from build123d import *

# Parameters (mm, degrees)
ESQUISSE1_W             = 100
ESQUISSE1_H             = 150
BOSS_EXTRU_1_DEPTH      = 100
ESQUISSE2_W             = 90
ESQUISSE2_H             = 140
ENL_V_MAT_EXTRU_1_DEPTH = 95
ESQUISSE4_W             = 40
ESQUISSE4_H             = 150
BOSS_EXTRU_2_DEPTH      = 10
ESQUISSE5_W             = 6
ESQUISSE5_H             = 150
ENL_V_MAT_EXTRU_2_DEPTH = 5
ESQUISSE7_W             = 40
ESQUISSE7_H             = 150
BOSS_EXTRU_3_DEPTH      = 10
ESQUISSE8_W             = 6
ESQUISSE8_H             = 150
ENL_V_MAT_EXTRU_3_DEPTH = 5
ESQUISSE9_W             = 5
ESQUISSE9_H             = 5
ENL_V_MAT_EXTRU_4_DEPTH = 121
ESQUISSE10_W            = 2.816855809
ESQUISSE10_H            = 20
BOSS_EXTRU_4_DEPTH      = 20
ESQUISSE11_R            = 4
ENL_V_MAT_EXTRU_5_DEPTH = 111


with BuildPart() as part:
    # Esquisse1 → Boss.-Extru.1 (new body)
    with BuildSketch(Plane.XY):
        with Locations((50, 75)):
            Rectangle(ESQUISSE1_W, ESQUISSE1_H)
    extrude(amount=BOSS_EXTRU_1_DEPTH)

    # Esquisse2 → Enlèv. mat.-Extru.1 (cut)
    with BuildSketch(Plane(origin=(0, 0, 0), x_dir=(-1, 0, 0), z_dir=(0, 0, -1))):
        with Locations((-50, 75)):
            Rectangle(ESQUISSE2_W, ESQUISSE2_H)
    extrude(amount=-ENL_V_MAT_EXTRU_1_DEPTH, mode=Mode.SUBTRACT)

    # Esquisse4 → Boss.-Extru.2 (add)
    with BuildSketch(Plane.ZY):
        with Locations((50, 75)):
            Rectangle(ESQUISSE4_W, ESQUISSE4_H)
    extrude(amount=BOSS_EXTRU_2_DEPTH)

    # Esquisse5 → Enlèv. mat.-Extru.2 (cut)
    with BuildSketch(Plane.ZY.offset(10)):
        with Locations((50, 75)):
            Rectangle(ESQUISSE5_W, ESQUISSE5_H)
    extrude(amount=-ENL_V_MAT_EXTRU_2_DEPTH, mode=Mode.SUBTRACT)

    # Esquisse7 → Boss.-Extru.3 (add)
    with BuildSketch(Plane(origin=(100, 0, 0), x_dir=(0, 0, -1), z_dir=(1, 0, 0))):
        with Locations((-50, 75)):
            Rectangle(ESQUISSE7_W, ESQUISSE7_H)
    extrude(amount=BOSS_EXTRU_3_DEPTH)

    # Esquisse8 → Enlèv. mat.-Extru.3 (cut)
    with BuildSketch(Plane(origin=(110, 0, 0), x_dir=(0, 0, -1), z_dir=(1, 0, 0))):
        with Locations((-50, 75)):
            Rectangle(ESQUISSE8_W, ESQUISSE8_H)
    extrude(amount=-ENL_V_MAT_EXTRU_3_DEPTH, mode=Mode.SUBTRACT)

    # Esquisse9 → Enlèv. mat.-Extru.4 (cut, through all)
    with BuildSketch(Plane(origin=(110, 0, 0), x_dir=(0, 0, -1), z_dir=(1, 0, 0))):
        with Locations((-38.25, 123.5)):
            Rectangle(ESQUISSE9_W, ESQUISSE9_H)
        with Locations((-60.75, 74.5)):
            Rectangle(ESQUISSE9_W, ESQUISSE9_H)
        with Locations((-38.25, 74.5)):
            Rectangle(ESQUISSE9_W, ESQUISSE9_H)
        with Locations((-60.75, 26.5)):
            Rectangle(ESQUISSE9_W, ESQUISSE9_H)
        with Locations((-60.75, 123.5)):
            Rectangle(ESQUISSE9_W, ESQUISSE9_H)
        with Locations((-38.25, 26.5)):
            Rectangle(ESQUISSE9_W, ESQUISSE9_H)
    extrude(amount=-ENL_V_MAT_EXTRU_4_DEPTH, mode=Mode.SUBTRACT)

    # Esquisse10 → Boss.-Extru.4 (add)
    with BuildSketch(Plane(origin=(0, 150, 0), x_dir=(1, 0, 0), z_dir=(0, 1, 0))):
        with Locations((98.591572095, -85)):
            Rectangle(ESQUISSE10_W, ESQUISSE10_H)
    extrude(amount=BOSS_EXTRU_4_DEPTH)

    # Esquisse11 → Enlèv. mat.-Extru.5 (cut, through all)
    with BuildSketch(Plane(origin=(100, 0, 0), x_dir=(0, 0, -1), z_dir=(1, 0, 0))):
        with Locations((-85, 160)):
            Circle(ESQUISSE11_R)
    extrude(amount=-ENL_V_MAT_EXTRU_5_DEPTH, mode=Mode.SUBTRACT)


solid = part.part
Can you work these out from the model? Positions are in its coordinate system, mm. A direction names the side the tool comes from. Give positions to 0.01 mm unless a question says otherwise; leave off trailing zeros. Loops run counter-clockwise (first coordinate to the right, second up) from the corner with the lowest first, then second, coordinate; pieces in that order, holes last. Notation, with made-up numbers: (-36.5, 10) - (-12.5, 10) arc R8 ccw to (-12.5, 16) - close; hole circle Ø8 at (47.5, 21). An arc over 180 degrees is marked (long way). Return JSON: item names as keys, results as strings.
1. For faces 1 (the face through (-2, 123, 40.75)), 2 (the face through (51, 145, 47)), 3 (the face through (-10, 76, 65)), which set-ups out of +Z, -Z, +X, -X, +Y, -Y let a thin tool reach every point of the face, with its end or its side?
Output values:
{"face 1": "+X, -X", "face 2": "-Z", "face 3": "+Z, -Z, -X, +Y, -Y"}
2. We'd pull the mould along Z, two halves only. Please class faces 4 (the face through (100, 74, 15)), 5 (the face through (103, 72, 38)): +Z half, -Z half, draft (parallel to the pull), parting line (faces both ways), or undercut.
Output values:
{"face 4": "draft", "face 5": "undercut"}
3. I'm going to push flat-ended pins straight in: pin 1 Ø1.5 at (x, y) = (91, 133.5) entering from -Z; pin 2 Ø2.5 at (x, y) = (108.5, 96) entering from +Z; pin 3 Ø5.5 at (x, z) = (-4, 61) entering from +Y. Where does each tip first touch, or does it pass through?
Output values:
{"pin 1": "stops at z = 95", "pin 2": "stops at z = 70", "pin 3": "stops at y = 150"}
4. If I drill on line 1 (Y direction, x = 23, z = 65); line 2 (X direction, y = 116.5, z = 45); line 3 (Y direction, x = 99, z = 85), over which ranges is the centre line in solid material (lowest first)?
Output values:
{"line 1": "y = 0 to 5, 145 to 150", "line 2": "x = -10 to 5, 95 to 110", "line 3": "y = 0 to 156, 164 to 170"}
5. I want a section at B-B on y = 160. Please give me the cut outline in (x, z), and give its area (3 significant figures).
Output values:
{"outline": "(97.18, 75) - (100, 75) - (100, 81) - (97.18, 81) - close; (97.18, 89) - (100, 89) - (100, 95) - (97.18, 95) - close", "area": "33.8 mm²"}
6. I want a section at D-D on y = 133. Please give me the cut outline in (x, z).
Output values:
{"outline": "(-10, 30) - (0, 30) - (0, 0) - (5, 0) - (5, 95) - (95, 95) - (95, 0) - (100, 0) - (100, 30) - (110, 30) - (110, 47) - (105, 47) - (105, 53) - (110, 53) - (110, 70) - (100, 70) - (100, 100) - (0, 100) - (0, 70) - (-10, 70) - (-10, 53) - (-5, 53) - (-5, 47) - (-10, 47) - close"}
7. I want a section at C-C on x = 74.5. Please give me the cut outline in (y, z).
Output values:
{"outline": "(0, 0) - (5, 0) - (5, 95) - (145, 95) - (145, 0) - (150, 0) - (150, 100) - (0, 100) - close"}
8. I want a section at A-A on z = 85. Please give me the cut outline in (x, y).
Output values:
{"outline": "(0, 0) - (100, 0) - (100, 156) - (97.18, 156) - (97.18, 150) - (0, 150) - close; (97.18, 164) - (100, 164) - (100, 170) - (97.18, 170) - close; hole (5, 5) - (95, 5) - (95, 145) - (5, 145) - close"}
